The listing builds one solid part. Answer for the finished solid, in the listing's coordinates (mm). A direction names the side the tool comes from. Give positions to 0.01 mm unless a question says otherwise; leave off trailing zeros. Loops run counter-clockwise (first coordinate to the right, second up) from the corner with the lowest first, then second, coordinate; pieces in that order, holes last. Notation, with made-up numbers: (-7.5, 38.25) - (41.5, 38.25) arc R27 cw to (41.5, 66.25) - close; hole circle Ø5 at (25.25, 55.25). An arc over 180 degrees is marked (long way). One line per item, written item: value. Start each with the question number.
from build123d import *

# Parameters (mm, degrees)
SKETCH1_W           = 200
SKETCH1_H           = 35
SKETCH1_R           = 3
BODY_DEPTH          = 4
SKETCH1_3_R         = 3
SKETCH1_3_R_2       = 1.5
SCREW_INSERTS_DEPTH = 2
SERVO_INSERT_DEPTH  = 38
SKETCH3_W           = 5
SKETCH3_H           = 3
WIRE_CHANNEL_DEPTH  = 10
SKETCH4_R           = 1.75
M2X4X3_5_DEPTH      = 6


with BuildPart() as part:
    # Sketch1 → Body (new body)
    with BuildSketch(Plane.XY):
        with Locations((100, 17.5)):
            Rectangle(SKETCH1_W, SKETCH1_H)
        with Locations((158, 30)):
            Circle(SKETCH1_R, mode=Mode.SUBTRACT)
        with Locations((42, 30)):
            Circle(SKETCH1_R, mode=Mode.SUBTRACT)
    extrude(amount=BODY_DEPTH)

    # Sketch1_3 → Screw Inserts (add)
    # profile 1 of 2: a face of its own
    with BuildSketch(Plane.XY):
        with Locations((42, 30)):
            Circle(SKETCH1_3_R)
        with Locations((42, 30)):
            Circle(SKETCH1_3_R_2, mode=Mode.SUBTRACT)
    # profile 2 of 2: a face of its own
    with BuildSketch(Plane.XY):
        with Locations((158, 30)):
            Circle(SKETCH1_3_R)
        with Locations((158, 30)):
            Circle(SKETCH1_3_R_2, mode=Mode.SUBTRACT)
    extrude(amount=SCREW_INSERTS_DEPTH)

    # Sketch2 → Servo Insert (add)
    with BuildSketch(Plane.XY.offset(4)):
        Polygon((88.75, 18), (83.25, 18), (83.25, 0), (116.75, 0), (116.75, 18), (111.25, 18), (111.25, 3), (88.75, 3), align=None)
    extrude(amount=SERVO_INSERT_DEPTH)

    # Sketch3 → Wire Channel (cut)
    with BuildSketch(Plane.XY.offset(42)):
        with Locations((114.25, 7.5)):
            Rectangle(SKETCH3_W, SKETCH3_H)
    extrude(amount=-WIRE_CHANNEL_DEPTH, mode=Mode.SUBTRACT)

    # Sketch4 → M2x4x3.5 (cut)
    with BuildSketch(Plane(origin=(0, 18, 0), x_dir=(1, 0, 0), z_dir=(0, 1, 0))):
        with Locations(Location((86, -36, 0), (0, 0, 180))):
            Circle(SKETCH4_R)
        with Locations((114, -36)):
            Circle(SKETCH4_R)
    extrude(amount=-M2X4X3_5_DEPTH, mode=Mode.SUBTRACT)


solid = part.part
1. A cutting plane is placed at C-C (z = 25). Determine the outline of the cut face in (x, y).
2. A cutting plane is placed at A-A (y = 16). Determine the outline of the cut face in (x, z).
3. A cutting plane is placed at B-B (x = 114). Determine the outline of the cut face in (y, z), plus the area to 3 significant figures.
4. Find the intervals of material crossed by L1, parallel to X at y = 12.5, z = 38; L2, parallel to Y at x = 158, z = 0.55; L3, parallel to Y at x = 42, z = 2.7, in increasing order. Write a range as [from, to].
5. For faces 1 (the flat face through (86, 12, 36)), 2 (the flat face through (88.75, 10, 23)), 3 (the flat face through (114, 9, 37)), 4 (the cylindrical face through (160.86, 30.9, 2.99)), 5 (the flat face through (0, 17, 2)), determine the directions among +Z, -Z, +X, -X, +Y, -Y from which every point of the face is accessible in a straight line to the end or side of a thin tool.
6. Determine the mould class of faces 6 (the flat face through (100, 0, 16)), 7 (the cylindrical face through (39, 30, 3)), 8 (the cylindrical face through (84.331, 15.042, 36.526)) for opening direction Y: released by +Y, released by -Y, zero draft, split by the parting line, or undercut.
7. Flat-ended cylindrical pins translate along their axes: pin 1 (1 mm diameter, centred on x = 114, z = 35.5, fed in from +Y); pin 2 (16.5 mm diameter, centred on y = 10, z = 28.5, fed in from +X); pin 3 (17.5 mm diameter, centred on x = 139, y = 15.5, fed in from +Z); pin 4 (1 mm diameter, centred on x = 167, y = 13.5, fed in from -Z). Find the tip coordinate at first contact, or state that the pin passes through.
8. A cutting plane is placed at D-D (x = 86). Determine the outline of the cut face in (y, z).
Results below:
1. outline: (83.25, 0) - (116.75, 0) - (116.75, 18) - (111.25, 18) - (111.25, 3) - (88.75, 3) - (88.75, 18) - (83.25, 18) - close
2. outline: (0, 0) - (200, 0) - (200, 4) - (116.75, 4) - (116.75, 42) - (111.25, 42) - (111.25, 4) - (88.75, 4) - (88.75, 42) - (83.25, 42) - (83.25, 4) - (0, 4) - close; hole circle Ø3.5 at (86, 36); hole circle Ø3.5 at (114, 36)
3. outline: (0, 0) - (35, 0) - (35, 4) - (18, 4) - (18, 34.25) - (12, 34.25) - (12, 37.75) - (18, 37.75) - (18, 42) - (9, 42) - (9, 32) - (6, 32) - (6, 42) - (0, 42) - close
3. area: 773 mm^2
4. L1: x = [83.25, 88.75], [111.25, 116.75]
4. L2: y = [0, 28.5], [31.5, 35]
4. L3: y = [0, 27], [33, 35]
5. face 1: +Y
5. face 2: +Z, +Y
5. face 3: +Z, +X
5. face 4: +Z
5. face 5: +Z, -Z, -X, +Y, -Y
6. face 6: released by -Y
6. face 7: undercut
6. face 8: zero draft
7. pin 1: stops at y = 12
7. pin 2: stops at x = 116.75
7. pin 3: stops at z = 4
7. pin 4: stops at z = 0
8. outline: (0, 0) - (35, 0) - (35, 4) - (18, 4) - (18, 34.25) - (12, 34.25) - (12, 37.75) - (18, 37.75) - (18, 42) - (0, 42) - close
